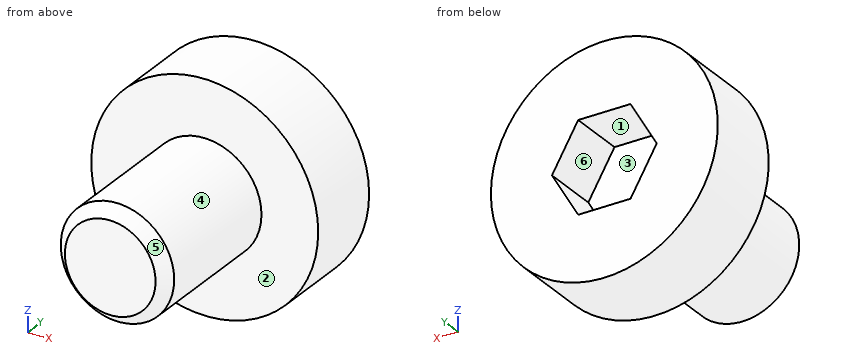
from build123d import *

# Parameters (mm, degrees)
F2_SIZE  = 2.54
F4_DEPTH = 12.7


with BuildPart() as f1:
    # F0 (on Top) → F1 (revolve)
    with BuildSketch(Plane.XY):
        Polygon((0, 50.8), (0, 0), (12.7, 0), (12.7, 33.02), (25.4, 33.02), (25.4, 50.8), align=None)
    revolve(axis=Axis((0, 25.4, 0), (0, 1, 0)))

    # F2
    f2_edges = [f1.edges().sort_by_distance(p)[0] for p in [
        (-12.7, 0, 0),
    ]]
    chamfer(f2_edges, length=F2_SIZE)

    # F3 (on face) → F4 (cut)
    with BuildSketch(Plane(origin=(0, 50.8, 0), x_dir=(-1, 0, 0), z_dir=(0, 1, 0))):
        Polygon((-5.865879, 10.16), (-11.731757, 0), (-5.865879, -10.16), (5.865879, -10.16), (11.731757, 0), (5.865879, 10.16), align=None)
    extrude(amount=-F4_DEPTH, mode=Mode.SUBTRACT)


solid = f1.part
Input: part model. Units: mm. Frame: model coordinates. Face numbers are marked on the shaded views. A direction names the side the tool comes from. Coordinates: 2 decimals unless noted, no trailing zeros. Order: outer loops, then holes, each group sorted by start corner. A loop starts at its lowest first (then second) coordinate and runs counter-clockwise, first axis right, second up.
1. Contact query for flat-ended pins moving along their axis: P1, Ø6, axis at x = 0.5, y = 44.5, coming from the -Z side; P2, Ø10, axis at x = -8.5, y = 26.5, coming from the -Z side; P3, Ø6, axis at x = -10, y = 6, coming from the -Z side. Output: stop coordinate, or through.
Checked values:
P1: stops at z = -25.4
P2: stops at z = -12.21
P3: stops at z = -10.6
2. Cut plane A-A, the plane y = 39.5. Return loops of the section in (x, z), plus the area to 3 significant figures.
Checked values:
outline: circle Ø50.8 at (0, 0); hole (-11.73, 0) - (-5.87, -10.16) - (5.87, -10.16) - (11.73, 0) - (5.87, 10.16) - (-5.87, 10.16) - close
area: 1,670 mm2
3. Draft query along Z for the marked faces 1, 2, 3 and 4. Return one class per face: +Z half, -Z half, draft (parallel to the pull), parting line (faces both ways), or undercut.
Checked values:
face 1: undercut
face 2: draft
face 3: undercut
face 4: parting line
4. Ray query, line 1 along Y through (x, z) = (1.5, 8); line 2 along Y through (x, z) = (-9, 13); line 3 along X through (y, z) = (39.5, 10). Return the intervals inside material, ascending.
Checked values:
line 1: y = 0 to 38.1
line 2: y = 33.02 to 50.8
line 3: x = -23.35 to -5.96, 5.96 to 23.35
5. Access query for the marked faces 5 and 6. Directions: +Z, -Z, +X, -X, +Y, -Y. A direction counts if a zero-diameter tool reaches every point of the face in a straight line with its end or side. Return the directions, or none.
Checked values:
face 5: -Y
face 6: +Y
6. Cut plane C-C, the plane y = 15.5. Return loops of the section in (x, z), plus the area to 3 significant figures.
Checked values:
outline: circle Ø25.4 at (0, 0)
area: 507 mm2
7. Cut plane B-B, the plane x = 0. Return loops of the section in (y, z), plus the area to 3 significant figures.
Checked values:
outline: (0, -10.16) - (2.54, -12.7) - (33.02, -12.7) - (33.02, -25.4) - (50.8, -25.4) - (50.8, -10.16) - (38.1, -10.16) - (38.1, 10.16) - (50.8, 10.16) - (50.8, 25.4) - (33.02, 25.4) - (33.02, 12.7) - (2.54, 12.7) - (0, 10.16) - close
area: 1,480 mm2
8. Cut plane D-D, the plane z = -19.5. Return loops of the section in (x, y).
Checked values:
outline: (-16.28, 33.02) - (16.28, 33.02) - (16.28, 50.8) - (-16.28, 50.8) - close
